Part model, mm, in its own coordinate system. Round coordinates to 2 decimals unless told otherwise and drop trailing zeros. Write each loop counter-clockwise with the first axis right and the second up, starting at its lowest first coordinate (ties: lowest second). Pieces come first, ordered by that corner, then holes.
from build123d import *

# Parameters (mm, degrees)
SKETCH1_W             = 127
SKETCH1_H             = 25.4
BOSS_EXTRUDE1_DEPTH   = 2.54
F_8_CLEARANCE_HOLE1_D = 4.4958
FILLET1_R             = 2.54


with BuildPart() as part:
    # Sketch1 → Boss-Extrude1 (new body)
    with BuildSketch(Plane(origin=(0, 0, 0), x_dir=(0, 0, -1), z_dir=(1, 0, 0))):
        with Locations((0, -11.049)):
            Rectangle(SKETCH1_W, SKETCH1_H)
    extrude(amount=BOSS_EXTRUDE1_DEPTH)

    # #8 Clearance Hole1 (through all)
    with Locations(Plane.ZY):
        with Locations((-50.8, -11.049), (-25.4, -11.049), (-38.1, -11.049), (0, -11.049), (25.4, -11.049), (50.8, -11.049), (-12.7, -11.049), (12.7, -11.049), (38.1, -11.049)):
            Hole(F_8_CLEARANCE_HOLE1_D / 2)

    # Fillet1
    fillet1_edges = [part.edges().sort_by_distance(p)[0] for p in [
        (1.27, -23.749, 63.5),
        (1.27, 1.651, 63.5),
        (1.27, 1.651, -63.5),
        (1.27, -23.749, -63.5),
    ]]
    fillet(fillet1_edges, radius=FILLET1_R)


solid = part.part
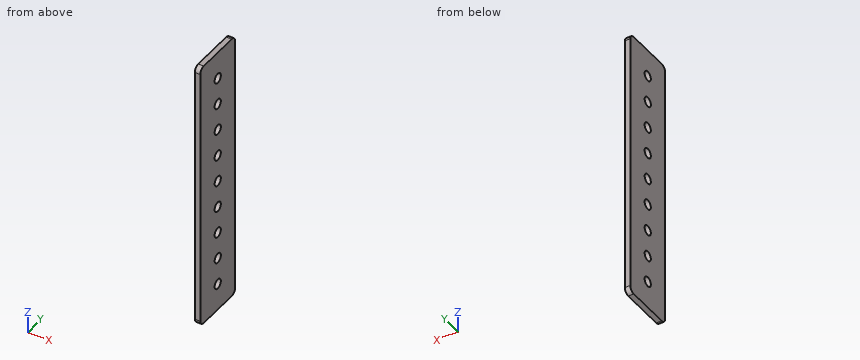
Q1. Wall check: line 1 (Y direction, x = 1.7, z = -38.1); line 2 (Y direction, x = 2.15, z = -52); line 3 (Z direction, x = 0.8, y = -21.5). Give the ranges that are in metal, low to high.
Q2. Drop flat-ended pins along their axis: P1, Ø4, axis at y = -11.049, z = 0, coming from the +X side; P2, Ø10, axis at y = -13, z = 24.5, coming from the +X side. Give the stop position or say it passes through.
Q3. Saw through at C-C, the plane z = 38. Write the cut outline in (x, y).
Q4. Saw through at A-A, the plane z = 0. Write the cut outline in (x, y).
Q5. Saw through at B-B, the plane x = 1.25. Give the number of separate pieces and of enclosed holes in the cut face, and give its area (3 significant figures).
Computed:
1. line 1: y = -23.75 to -13.3, -8.8 to 1.65
1. line 2: y = -23.75 to -12.95, -9.15 to 1.65
1. line 3: z = -63.48 to 63.48
2. P1: passes through
2. P2: stops at x = 2.54
3. outline: (0, -23.75) - (2.54, -23.75) - (2.54, -13.29) - (0, -13.29) - close; (0, -8.8) - (2.54, -8.8) - (2.54, 1.65) - (0, 1.65) - close
4. outline: (0, -23.75) - (2.54, -23.75) - (2.54, -13.3) - (0, -13.3) - close; (0, -8.8) - (2.54, -8.8) - (2.54, 1.65) - (0, 1.65) - close
5. separate pieces: 1
5. enclosed holes: 9
5. area: 3,080 mm2
